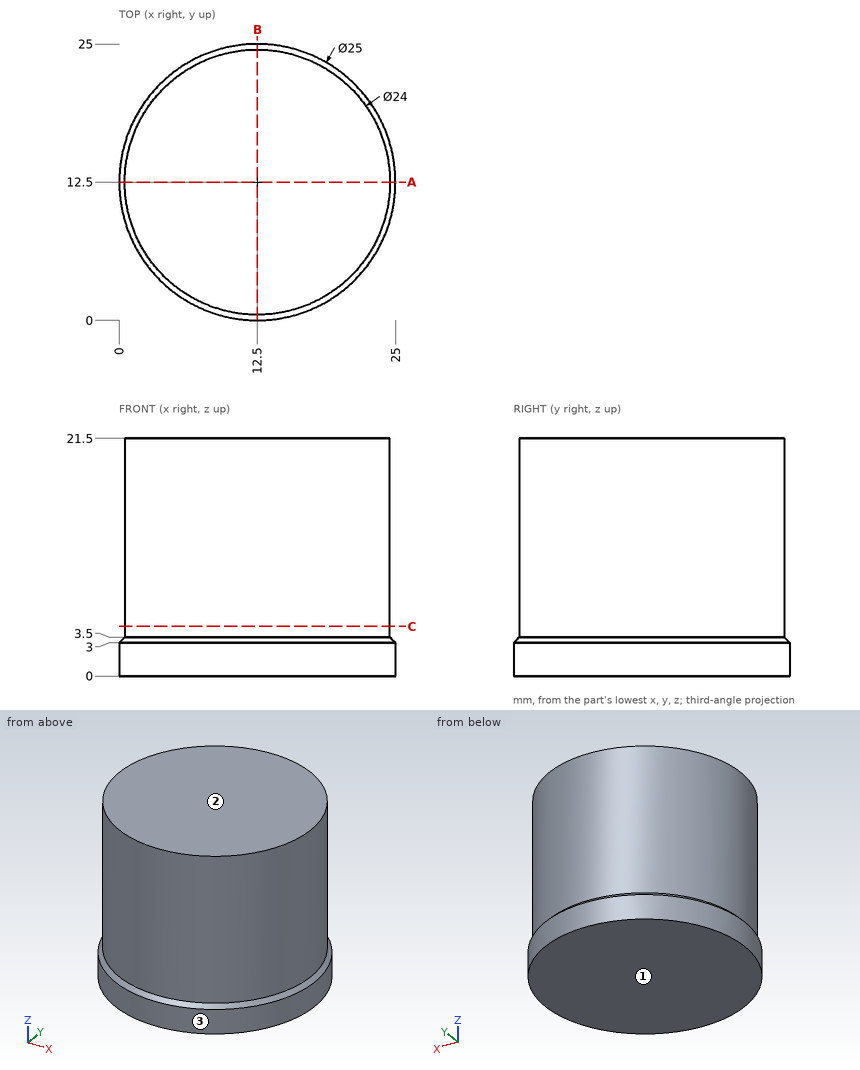
Geometry check sheet. Reference: drawing and pictorial views, mm from the part's lowest x, y, z. Round coordinates to 2 decimals unless told otherwise and drop trailing zeros. Loops run counter-clockwise (first coordinate to the right, second up) from the corner with the lowest first, then second, coordinate; pieces in that order, holes last.
1. Mould release check, pull along Z, two halves, no side actions. Record for the marked faces 1, 2 and 3: released by +Z, released by -Z, zero draft, split by the parting line, or undercut.
2. Sectioned sample at A-A on y = 12.5. Record the boundary of the cut face in (x, z), and give its area (3 significant figures).
3. Sectioned sample at C-C on z = 4.5. Record the boundary of the cut face in (x, y).
4. Gauge pin test, flat ends, axial feed: pin 1 Ø3 at (x, z) = (22.5, 11.5) entering from +Y; pin 2 Ø6 at (x, z) = (19.5, 4) entering from -Y; pin 3 Ø6 at (x, z) = (5.5, 9) entering from -Y. Record the tip position at first contact, or that the pin passes through.
5. Scan lines: probe 1 along Y at (x, z) = (12.5, 9.25); probe 2 along X at (y, z) = (4.25, 2.5); probe 3 along Y at (x, z) = (10, 11.5). Record each from-to range of solid material in increasing order.
Recorded:
1. face 1: released by -Z
1. face 2: released by +Z
1. face 3: zero draft
2. outline: (0, 0) - (25, 0) - (25, 3) - (24.5, 3.5) - (24.5, 21.5) - (0.5, 21.5) - (0.5, 3.5) - (0, 3) - close
2. area: 519 mm2
3. outline: circle Ø24 at (12.5, 12.5)
4. pin 1: stops at y = 20.97
4. pin 2: stops at y = 0.72
4. pin 3: stops at y = 1.19
5. probe 1: y = 0.5 to 24.5
5. probe 2: x = 3.11 to 21.89
5. probe 3: y = 0.76 to 24.24
